Job drawing, mm, ordinate dimensions from the low corner. One solid piece. A direction names the side the tool comes from. Coordinates: 2 decimals unless noted, no trailing zeros. Write each loop counter-clockwise with the first axis right and the second up, starting at its lowest first coordinate (ties: lowest second). Pieces come first, ordered by that corner, then holes.
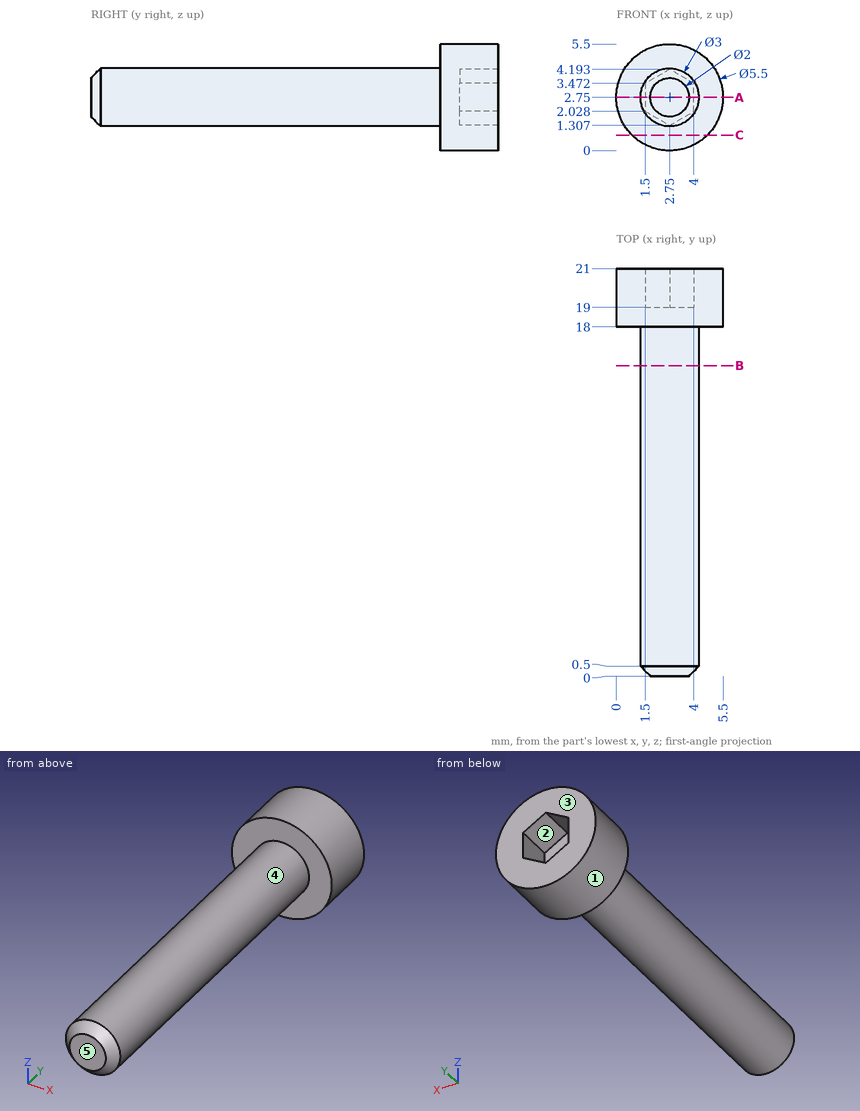
1. Saw through at C-C on z = 0.8. List the corners of the cut face in (x, y), plus the area to 3 significant figures.
Computed values:
outline: (0.81, 18) - (4.69, 18) - (4.69, 21) - (0.81, 21) - close
area: 11.6 mm2
2. 3-axis set-ups, long thin cutter, end or side, ignore diameter. For the marked faces 4 and 5: which of +Z, -Z, +X, -X, +Y, -Y reach the whole face in a straight line?
Computed values:
face 4: -Y
face 5: +Z, -Z, +X, -X, -Y
3. Probe line 1 along Y through (x, z) = (2.65, 1.9); line 2 along Y through (x, z) = (4.7, 2.7); line 3 along X through (y, z) = (7.5, 2.8). List the from-to ranges inside material, lowest first.
Computed values:
line 1: y = 0 to 19
line 2: y = 18 to 21
line 3: x = 1.25 to 4.25
4. Mould opens along X. For the marked faces 1, 2 and 3 say: +X half, -X half, draft (parallel to the pull), parting line (faces both ways), or undercut.
Computed values:
face 1: parting line
face 2: undercut
face 3: draft
5. Flat gauge pins, fed straight in: pin 1 (0.8 mm diameter, centred on x = 2.5, z = 3, fed in from +Y); pin 2 (3 mm diameter, centred on x = 4, y = 2, fed in from -Z); pin 3 (3 mm diameter, centred on y = 6.5, z = 0.5, fed in from -X). Where does each tip first touch, or does it go through?
Computed values:
pin 1: stops at y = 19
pin 2: stops at z = 1.25
pin 3: stops at x = 1.45
6. Saw through at B-B on y = 16. List the corners of the cut face in (x, z).
Computed values:
outline: circle Ø3 at (2.75, 2.75)
7. Saw through at A-A on z = 2.75. List the corners of the cut face in (x, y).
Computed values:
outline: (0, 18) - (1.25, 18) - (1.25, 0.5) - (1.75, 0) - (3.75, 0) - (4.25, 0.5) - (4.25, 18) - (5.5, 18) - (5.5, 21) - (4, 21) - (4, 19) - (1.5, 19) - (1.5, 21) - (0, 21) - close
